Autodesk Inventor part; units mm, degrees
ref_plane "Work Plane1" through (-49.846, -23.6605, 0) normal (0, 0, 1) x (1, 0, 0)
ref_plane "YZ Plane" through (0, 0, 0) normal (1, 0, 0) x (0, 1, 0)
ref_plane "XZ Plane" through (0, 0, 0) normal (0, 1, 0) x (-1, 0, 0)
sketch "Sketch2" plane through (0, 0, 0) normal (1, 0, 0) x (0, 1, 0)
  line L0 (-23.6605, 0) -> (-23.6605, 2.54)
  line L1 (-23.6605, 2.54) -> (-17.3105, 2.54)
  line L2 (-17.3105, 2.54) -> (-4.721, 73.9386)
  line L3 (10.5271, 0) -> (9.3929, 0)
  line L4 (-4.721, 73.9386) -> (-2.2195, 73.4975)
  line L5 (-4.721, 73.9386) -> (-2.181, 73.9386) construction
  line L6 (-23.3526, 2.54) -> (0, 2.54)
  line L7 (0, 2.54) -> (0, 0)
  line L8 (0, 0) -> (-23.3526, 0)
  line L9 (-23.3526, 0) -> (-23.3526, 2.54)
  line L10 (-2.2195, 73.4975) -> (-14.7313, 2.54)
  point P0 (23.6605, 0)
  point P1 (-4.0951, 0)
  point P2 (-6.6351, 0)
  dimension "d2" = 2.54
  dimension "d3" = 6.35
  dimension "d5" = 100
  dimension "d6" = 2.54
  dimension "d7" = 10
  dimension "d9" = 72.5
extrude "Extrusion1" add sketch "Sketch2" along normal mid plane 55
sketch "Sketch3" plane through (0, 0, 0) normal (1, 0, 0) x (0, 1, 0)
  line L0 (-2.2195, 73.4975) -> (-2.2195, 2.54)
  line L1 (0, 2.54) -> (-14.7313, 2.54)
  line L2 (-14.7313, 2.54) -> (-2.2195, 73.4975)
  line L3 (-2.2195, 73.4975) -> (-14.7313, 2.54)
  line L4 (-2.2195, 73.4975) -> (0, 73.4975)
  line L5 (0, 73.4975) -> (-2.2195, 2.54)
  point P0 (0, 0)
extrude "Extrusion2" add sketch "Sketch3" along normal mid plane 6.35
sketch "Sketch4" plane through (-27.5, -17.3105, 2.54) normal (0, -0.9848078, 0.1736482) x (1, 0, 0)
  line L0 (2.5, 71.4739) -> (2.5, 1.4739) construction
  line L1 (2.5, 1.4739) -> (52.5, 1.4739) construction
  line L2 (52.5, 1.4739) -> (52.5, 71.4739) construction
  line L3 (52.5, 71.4739) -> (2.5, 71.4739) construction
  line L4 (2.5, 71.4739) -> (52.5, 1.4739) construction
  line L5 (2.5, 1.4739) -> (52.5, 71.4739) construction
  line L6 (55, 0.4479) -> (55, 72.5)
  line L7 (2.5, 71.4739) -> (72.5, 71.4739) construction
  line L8 (55, 36.4739) -> (55, 71.4739)
  line L9 (55, 36.4739) -> (55, 1.4739)
  line L10 (55, 72.5) -> (55, 0)
  line L11 (55, 55.3) -> (52.5, 55.3)
  line L12 (55, 17.2) -> (52.5, 17.2)
  line L13 (0, 0) -> (0, 72.5)
  line L14 (0, 36.4739) -> (0, 71.4739)
  line L15 (0, 36.4739) -> (0, 1.7269)
  line L16 (0, 0.4479) -> (0, 3.0059)
  line L17 (0, 17.2) -> (2.5, 17.2)
  line L18 (0, 55.3) -> (2.5, 55.3)
  circle A0 centre (55, 55.3) radius 2.5
  circle A1 centre (55, 17.2) radius 2.5
  circle A2 centre (0, 55.3) radius 2.5
  circle A3 centre (0, 17.2) radius 2.5
  point P0 (27.5, 0.5045)
  point P1 (27.5, 36.4739)
  point P2 (27.5, 36.4739)
  point P3 (27.5, 36.4739)
  point P4 (55, 36.25)
  point P5 (55, 36.25)
  point P6 (0, 52.8)
  point P7 (0, 57.8)
  point P8 (0, 14.7)
  point P9 (0, 19.7)
  point P10 (55, 14.7)
  point P11 (55, 19.7)
  point P12 (55, 52.8)
  point P13 (55, 57.8)
  dimension "d14" = 70
  dimension "d15" = 90
  dimension "d16" = 50
  dimension "d17" = 19.05
  dimension "d18" = 19.05
extrude "Extrusion3" cut sketch "Sketch4" against normal through all contours A1 L12 L6 | L12 A1 L6 | A0 L11 L6 | L11 A0 L6 | L13 L17 A3 | L13 A3 L17 | L13 L18 A2 | L13 A2 L18
sketch "Sketch5" plane through (-27.5, 0, 2.54) normal (0, 0, 1) x (1, 0, 0)
  line L0 (64.0804, -22.4444) -> (30.0297, 6.1276)
  line L1 (-9.0804, -22.4444) -> (24.9703, 6.1276)
  line L2 (30.0297, 6.1276) -> (24.9703, 6.1276)
  line L3 (0, 0) -> (55, 0)
  line L4 (37.3323, 0) -> (17.6677, 0)
  point P0 (27.5, 0)
ref_plane "Work Plane1" through (-49.846, -23.6605, 0) normal (0, 0, 1) x (1, 0, 0)
extrude "Extrusion4" add sketch "Sketch5" against normal up to surface (2.54 mm away)
chamfer "Chamfer1" distance 12.7 angle 45 2 edges at (-27.5, 0, 1.27) (27.5, 0, 1.27)
sketch "Sketch6" plane through (-27.5, 0, 0) normal (-1, 0, 0) x (0, 0, 1)
  line L0 (73.9386, -4.721) -> (73.4975, -2.2195)
  line L1 (73.9386, -4.721) -> (75.3954, -6.8016)
  line L2 (73.9386, -4.721) -> (76.4786, -4.721) construction
  line L3 (75.3954, -6.8016) -> (75.3954, 0)
  line L4 (75.3954, 0) -> (73.4975, 0)
  line L5 (73.4975, 0) -> (73.4975, -2.2195)
  line L6 (54.0968, -5.6404) -> (59.0208, -4.7722)
  line L7 (73.4975, 0) -> (59.0208, -4.7722)
  line L8 (59.0208, -4.7722) -> (73.4975, -2.2195)
  line L9 (75.3954, -6.8016) -> (77.9354, -6.8016)
  line L10 (77.9354, -6.8016) -> (77.9354, 0)
  line L11 (77.9354, 0) -> (75.3954, 0)
  line L12 (75.3954, 0) -> (75.3954, -6.8016)
  point P0 (0, 0)
  dimension "d26" = 2.54
  dimension "d27" = 55
  dimension "d30" = 2.54
extrude "Extrusion5" add sketch "Sketch6" against normal up to surface (55 mm away)
sketch "Sketch7" plane through (-27.5, -14.7313, 2.54) normal (0, 0, 1) x (1, 0, 0)
  line L0 (12.7, 14.7313) -> (17.6677, 14.7313) construction
  line L1 (37.3323, 14.7313) -> (17.6677, 14.7313) construction
  line L2 (27.5, 14.7313) -> (27.5, 20.8588) construction
  line L3 (30.0297, 20.8588) -> (24.9703, 20.8588) construction
  line L4 (0, -2.5792) -> (55, -2.5792) construction
  line L5 (0, 2.0313) -> (0, -8.6214) construction
  line L6 (55, -2.5792) -> (0, -8.6214) construction
  line L7 (0, -8.6214) -> (0, -2.5792) construction
  line L8 (0, -8.6214) -> (55, -8.6214) construction
  line L9 (55, -8.6214) -> (0, -2.5792) construction
  line L10 (55, -8.6214) -> (55, 2.0313) construction
  line L11 (55, -5.6003) -> (0, -5.6003) construction
  point P0 (27.5, 16.8588)
  point P1 (40.2, -5.6003)
  point P2 (14.8, -5.6003)
  point P3 (27.5, -5.6003)
  point P4 (27.5, -5.6003)
  dimension "d31" = 4
  dimension "d39" = 12.7
  dimension "d40" = 12.7
hole "Hole1" at (0, 2.1276, 2.54) at (12.7, -20.3315, 2.54) at (-12.7, -20.3315, 2.54) direction (0, 0, -1) diameter 4 depth 5.8
properties part number "BreadboardHolderv1"
Here's how the part is built. I have some questions about the finished solid (model axes, mm). A direction names the side the tool comes from. Give positions to 0.01 mm unless a question says otherwise; leave off trailing zeros. Write each loop counter-clockwise with the first axis right and the second up, starting at its lowest first coordinate (ties: lowest second). Pieces come first, ordered by that corner, then holes. Notation, with made-up numbers: (12.25, 82) -> (62.25, 82) arc R29 ccw to (62.25, 112) -> close; hole circle Ø11 at (56, 27). An arc over 180 degrees is marked (long way). Use one line per item in the form item = value. Start each with the question number.
1. Will these pins go through, and if not, where does the flat tip stop? pin 1 Ø3 at (x, z) = (11.5, 1.5) entering from +Y; pin 2 Ø3 at (x, y) = (11.5, -21.5) entering from +Z; pin 3 Ø4 at (x, y) = (11.5, -10.5) entering from -Z; pin 4 Ø8 at (x, z) = (-12, 56.5) entering from -Y.
2. On a 3-axis mill with a long thin cutter (end or side, diameter ignored), from which of +Z, -Z, +X, -X, +Y, -Y can I reach the whole of each face in a straight line? I mean faces 1 (the face through (-21.1, -6.3, 1.3)), 2 (the face through (15.167, -2.353, 66.36)), 3 (the face through (-3.175, -6, 31)), 4 (the face through (-12, 0, 1)), 5 (the face through (0, -12, 0)). Say none if no direction works.
3. Imagine slicing it at D-D on z = 65. List the corners of the cut face in (x, y) for me (3 decimals).
4. Imagine slicing it at A-A on x = 0. List the corners of the cut face in (y, z) for me.
5. Thinking about a two-plate mould opening in X: for faces 6 (the face through (27.5, -4, 71)), 7 (the face through (-11.483, -18.744, 1.252)), 8 (the face through (-27.5, -16, 7)), which applies, +X half, -X half, draft (parallel to the pull), parting line (faces both ways), or undercut?
6. Imagine slicing it at B-B on x = 18. List the corners of the cut face in (y, z) for me.
7. Imagine slicing it at C-C on y = -19.5. List the corners of the cut face in (x, z) for me.
8. If I drill on L1, parallel to Y at x = -12.7, z = 1.25; L2, parallel to Y at x = 0, z = 1.65; L3, parallel to X at y = -8.75, z = 30.5 (3 decimals), over which ranges is the centre line in solid material (lowest first)?
Entries:
q1.pin_1 = 0
q1.pin_2 = 2.54
q1.pin_3 = 0
q1.pin_4 = -8.5
q2.face_1 = -Z, -X, +Y
q2.face_2 = +X, +Y
q2.face_3 = -X, +Y
q2.face_4 = +Z, -Z, -X, +Y
q2.face_5 = -Z, +X, -X, +Y, -Y
q3.outline = (-27.5, -6.297) -> (27.5, -6.297) -> (27.5, -2.801) -> (3.175, -2.801) -> (3.175, -0.266) -> (-3.175, -0.266) -> (-3.175, -2.801) -> (-27.5, -2.801) -> close
q4.outline = (-23.35, 0) -> (0.13, 0) -> (0.13, 2.54) -> (-2.22, 2.54) -> (0, 73.5) -> (0, 77.94) -> (-6.8, 77.94) -> (-6.8, 75.4) -> (-4.72, 73.94) -> (-17.31, 2.54) -> (-23.35, 2.54) -> close; (4.13, 0) -> (6.13, 0) -> (6.13, 2.54) -> (4.13, 2.54) -> close
q5.face_6 = +X half
q5.face_7 = undercut
q5.face_8 = -X half
q6.outline = (-23.35, 0) -> (-3.2, 0) -> (-3.2, 2.54) -> (-14.73, 2.54) -> (-4.77, 59.02) -> (0, 73.5) -> (0, 77.94) -> (-6.8, 77.94) -> (-6.8, 75.4) -> (-4.72, 73.94) -> (-17.31, 2.54) -> (-23.35, 2.54) -> close
q7.outline = (-27.5, 0) -> (-14.52, 0) -> (-14.52, 2.54) -> (-27.5, 2.54) -> close; (-10.88, 0) -> (10.88, 0) -> (10.88, 2.54) -> (-10.88, 2.54) -> close; (14.52, 0) -> (27.5, 0) -> (27.5, 2.54) -> (14.52, 2.54) -> close
q8.L1 = -23.35 to -22.33, -18.33 to 0
q8.L2 = -23.35 to 0.13, 4.13 to 6.13
q8.L3 = -3.175 to 3.175
